Geometry check sheet. Reference: the model listing, model coordinates, mm. Face numbers are marked on the shaded views. Coordinates: 2 decimals unless noted, no trailing zeros. Write each loop counter-clockwise with the first axis right and the second up, starting at its lowest first coordinate (ties: lowest second). Pieces come first, ordered by that corner, then holes. Notation, with made-up numbers: M -27,-4 L 3,-4 A19 ccw 3,31 Z; hole C 7.25,62 d6. An arc over 180 degrees is marked long. Put each result on its own line as item: value. Start each with the question number.
1) Mould release check, pull along X, two halves, no side actions. Record for the marked faces 1 and 2: released by +X, released by -X, zero draft, split by the parting line, or undercut.
2) Cross-section at A-A on z = 7. Record the cut outline in (x, y), plus the area to 3 significant figures.
3) Scan lines: line 1 along Y through (x, z) = (0, 23.5); line 2 along X through (y, z) = (0, 66.4). Record each from-to range of solid material in increasing order.
4) Gauge pin test, flat ends, axial feed: pin 1 (2 mm diameter, centred on x = -3, z = 7.5, fed in from -Y); pin 2 (1 mm diameter, centred on y = -1, z = 13, fed in from -X); pin 3 (6 mm diameter, centred on x = -3, z = 46, fed in from -Y); pin 4 (1 mm diameter, centred on x = 0.5, y = 1.5, fed in from +Z). Record the tip position at first contact, or that the pin passes through.
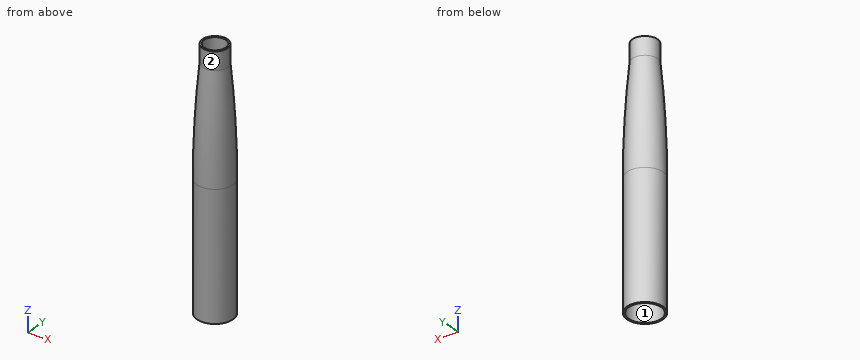
Autodesk Inventor part; units mm, degrees
ref_plane "YZ Plane" through (0, 0, 0) normal (1, 0, 0) x (0, 1, 0)
ref_plane "XZ Plane" through (0, 0, 0) normal (0, 1, 0) x (-1, 0, 0)
sketch "Sketch1" plane through (0, 0, 0) normal (0, 0, 1) x (1, 0, 0)
  circle A0 centre (0, 0) radius 4.5
  circle A1 centre (0, 0) radius 5
  line L0 (0, 0) -> (0, -5)
  dimension "d0" = 9
  dimension "d1" = 0.5
ref_plane "Work Plane1" through (0, 0, 35) normal (0, 0, 1) x (1, 0, 0)
ref_plane "Work Plane2" through (0, 0, 65) normal (0, 0, 1) x (1, 0, 0)
sketch "Sketch3" plane through (0, 0, 65) normal (0, 0, 1) x (1, 0, 0)
  circle A0 centre (0, 0) radius 3
  circle A1 centre (0, 0) radius 3.5
  line L0 (0, 0) -> (0, -3.5)
  dimension "d4" = 0.5
  dimension "d5" = 6
sketch "Sketch2" plane through (0, 0, 35) normal (0, 0, 1) x (1, 0, 0)
  circle A0 centre (0, 0) radius 5
  circle A1 centre (0, 0) radius 4.5
  line L0 (0, 0) -> (0, -5)
ref_plane "Work Plane3" through (0, 0, 0) normal (-1, 0, 0) x (0, -1, 0)
sketch "Sketch4" plane through (0, 0, 0) normal (-1, 0, 0) x (0, -1, 0)
  line L0 (5, 35) -> (5, 0)
  line L1 (5, 0) -> (4.5, 0)
  line L2 (4.5, 0) -> (4.5, 35)
  arc A0 (5, 35) -> (3.5, 65) centre (-295.75, 35) ccw
  line L3 (5, 0) -> (-5, 0)
  line L4 (4.5, 0) -> (-4.5, 0)
  line L5 (0, 0) -> (5, 0)
  line L6 (5, 35) -> (-5, 35)
  line L7 (0, 35) -> (5, 35)
  line L8 (4.5, 35) -> (-4.5, 35)
  line L9 (0, 65) -> (3.5, 65)
  line L10 (3.5, 65) -> (-3.5, 65)
  line L11 (3, 65) -> (-3, 65)
  line L12 (3.5, 65) -> (3, 65)
  arc A1 (4.5, 35) -> (3, 65) centre (-296.25, 35) ccw
  line L13 (0, 65) -> (0, 0)
revolve "Revolution2" add sketch "Sketch4" angle 360 about axis through (0, 0, 65) along (0, 0, -1) contours L6 A1 L9 A0 | L0 L1 L2 L6
sketch "Sketch5" plane through (0, 0, 65) normal (0, 0, 1) x (1, 0, 0)
  circle A0 centre (0, 0) radius 3.5
  circle A1 centre (0, 0) radius 2
  circle A2 centre (0, 0) radius 3
  dimension "d21" = 4
extrude "Extrusion1" add sketch "Sketch5" along normal blind 5 contours A0
properties part number "Hand"
Answer key:
1. face 1: undercut
1. face 2: split by the parting line
2. outline: C 0,0 d10; hole C 0,0 d9
2. area: 14.9 mm²
3. line 1: y = -5 to -4.5, 4.5 to 5
3. line 2: x = -3.5 to -3, 3 to 3.5
4. pin 1: stops at y = -4.58
4. pin 2: stops at x = -4.97
4. pin 3: stops at y = -4.83
4. pin 4: passes through
